```python
from build123d import *

# Parameters (mm, degrees)
BOSS_EXTRUDE1_DEPTH = 6
SKETCH2_W           = 15
SKETCH2_H           = 6
CUT_EXTRUDE1_DEPTH  = 10
FILLET1_R           = 5


with BuildPart() as part:
    # Sketch1 → Boss-Extrude1 (new body)
    with BuildSketch(Plane.XY):
        with BuildLine():
            Line((105.001506242, -129.791901429), (120.001506242, -129.791901429))
            Line((120.001506242, -129.791901429), (120.001506242, 0))
            ThreePointArc((120.001506242, 0), (91.250753121, 28.750753121), (62.5, 0))
            ThreePointArc((62.5, 0), (15.310848117, -60.595609824), (-54.998493758, -29.688645714))
            Line((-54.998493758, -29.688645714), (-54.998493758, -129.791901429))
            Line((-54.998493758, -129.791901429), (-54.998493758, -135.791901429))
            Line((-54.998493758, -135.791901429), (-9.998493758, -135.791901429))
            Line((-9.998493758, -135.791901429), (-9.998493758, -129.791901429))
            Line((-9.998493758, -129.791901429), (60.001506242, -129.791901429))
            Line((60.001506242, -129.791901429), (60.001506242, -135.791901429))
            Line((60.001506242, -135.791901429), (105.001506242, -135.791901429))
            Line((105.001506242, -135.791901429), (105.001506242, -129.791901429))
        make_face()
    extrude(amount=BOSS_EXTRUDE1_DEPTH)

    # Sketch2 → Cut-Extrude1 (cut)
    with BuildSketch(Plane.XY.offset(6)):
        with Locations((65.501506242, -86.791901429)):
            Rectangle(SKETCH2_W, SKETCH2_H)
        with Locations((100.501506242, -86.791901429)):
            Rectangle(SKETCH2_W, SKETCH2_H)
    extrude(amount=-CUT_EXTRUDE1_DEPTH, mode=Mode.SUBTRACT)

    # Fillet1
    fillet1_edges = [part.edges().sort_by_distance(p)[0] for p in [
        (-54.998493758, -29.688645714, 3),
    ]]
    fillet(fillet1_edges, radius=FILLET1_R)


solid = part.part
```
The model under review builds one solid part; all positions refer to its coordinate system, in mm. A direction names the side the tool comes from. Round coordinates to 2 decimals unless told otherwise and drop trailing zeros. Loops run counter-clockwise (first coordinate to the right, second up) from the corner with the lowest first, then second, coordinate; pieces in that order, holes last. Notation, with made-up numbers: M 31.5,61.25 L 84.5,61.25 A27 ccw 84.5,94.25 Z; hole C 35.25,53 d5. An arc over 180 degrees is marked long. Put each result on its own line as item: value.
Q1. Consider section B-B, the plane z = 3.35. Give the boundary of the cut face in (x, y).
Result set:
outline: M -55,-135.79 L -10,-135.79 L -10,-129.79 L 60,-129.79 L 60,-135.79 L 105,-135.79 L 105,-129.79 L 120,-129.79 L 120,0 A28.75 ccw 62.5,0 A62.5 cw -46.29,-41.99 A5 ccw -55,-45.35 Z; hole M 58,-89.79 L 73,-89.79 L 73,-83.79 L 58,-83.79 Z; hole M 93,-89.79 L 108,-89.79 L 108,-83.79 L 93,-83.79 Z
Q2. To check wall thickness, follow L1, parallel to X at y = -48, z = 3.25; L2, parallel to Y at x = 96, z = 3.2; L3, parallel to Y at x = 102.5, z = 5.15. State the ranges of each line that lie inside material, in increasing order.
Result set:
L1: x = -55 to -40.03, 40.03 to 120
L2: y = -135.79 to -89.79, -83.79 to 28.36
L3: y = -135.79 to -89.79, -83.79 to 26.46
Q3. Consider section C-C, the plane x = 1.5. Give the boundary of the cut face in (y, z), then the cut area to 3 significant figures.
Result set:
outline: M -129.79,0 L -62.48,0 L -62.48,6 L -129.79,6 Z
area: 404 mm²
Q4. Mouldability with a two-part tool opening along Y and no side actions: class faces 6 (the flat face through (112, -129.792, 3)), 7 (the flat face through (51, -71, 0)), 8 (the flat face through (100, -89.792, 3)), 9 (the cylindrical face through (23.48, -57.92, 2.96)) as released by +Y, released by -Y, zero draft, split by the parting line, or undercut.
Result set:
face 6: released by -Y
face 7: zero draft
face 8: undercut
face 9: released by +Y
Q5. Consider section A-A, the plane y = -57. Give the boundary of the cut face in (x, z), then the cut area to 3 significant figures.
Result set:
outline: M -55,0 L -25.64,0 L -25.64,6 L -55,6 Z; M 25.64,0 L 120,0 L 120,6 L 25.64,6 Z
area: 742 mm²
Q6. Consider section D-D, the plane y = -13. Give the boundary of the cut face in (x, z).
Result set:
outline: M 61.13,0 L 120,0 L 120,6 L 61.13,6 Z
Q7. Machinability: for faces 1 (the flat face through (65, -89.792, 3)), 2 (the flat face through (51, -71, 6)), 3 (the flat face through (82, -135.792, 3)), 4 (the flat face through (105.002, -133, 3)), 5 (the flat face through (-9.998, -133, 3)), which of the approach directions +Z, -Z, +X, -X, +Y, -Y give a long, thin tool a straight path to every point of the face, cutting with its end or side? Answer none if there is none.
Result set:
face 1: +Z, -Z
face 2: +Z, +X, -X, +Y, -Y
face 3: +Z, -Z, +X, -X, -Y
face 4: +Z, -Z, +X, -Y
face 5: +Z, -Z, -Y
Q8. For pin 1 (3 mm diameter, centred on x = 67.5, z = 4.5, fed in from +Y); pin 2 (1 mm diameter, centred on x = 29, z = 2, fed in from +Y); pin 3 (1.8 mm diameter, centred on y = -132, z = 4, fed in from +X), all flat-tipped, find the tip position at first contact; note any pin that passes through.
Result set:
pin 1: stops at y = 18.21
pin 2: stops at y = -55.1
pin 3: stops at x = 105
